```python
from build123d import *

# Parameters (mm, degrees)
BOSS_EXTRUDE1_DEPTH = 12.7
CUT_EXTRUDE1_DEPTH  = 25.4
CUT_EXTRUDE2_DEPTH  = 25.4
FILLET1_R           = 8.89
SKETCH4_R           = 2.54
CUT_EXTRUDE3_DEPTH  = 25.4


with BuildPart() as part:
    # Sketch1 → Boss-Extrude1 (new, symmetric)
    with BuildSketch(Plane.XY):
        Polygon((-19.05, 0), (19.05, 0), (19.05, -1.5875), (0, -3.175), (0, -1.5875), (-19.05, -1.5875), align=None)
    extrude(amount=BOSS_EXTRUDE1_DEPTH, both=True)

    # Sketch2 → Cut-Extrude1 (cut)
    with BuildSketch(Plane(origin=(0, 0, 0), x_dir=(1, 0, 0), z_dir=(0, 1, 0))):
        Polygon((0, 12.7), (19.05, 10.16), (19.05, 12.7), align=None)
    cut_extrude1 = extrude(amount=-CUT_EXTRUDE1_DEPTH, mode=Mode.SUBTRACT)

    # Mirror1: Cut-Extrude1 across plane
    add(cut_extrude1.mirror(Plane.XY), mode=Mode.SUBTRACT)

    # Sketch3 → Cut-Extrude2 (cut)
    with BuildSketch(Plane(origin=(0, 0, 0), x_dir=(1, 0, 0), z_dir=(0, 1, 0))):
        Polygon((0, 12.7), (-19.05, 7.62), (-19.05, 12.7), align=None)
    cut_extrude2 = extrude(amount=-CUT_EXTRUDE2_DEPTH, mode=Mode.SUBTRACT)

    # Mirror2: Cut-Extrude2 across plane
    add(cut_extrude2.mirror(Plane.XY), mode=Mode.SUBTRACT)

    # Fillet1
    fillet1_edges = [part.edges().sort_by_distance(p)[0] for p in [
        (-19.05, -0.79375, -7.62),
        (-19.05, -0.79375, 7.62),
    ]]
    fillet(fillet1_edges, radius=FILLET1_R)

    # Sketch4 → Cut-Extrude3 (cut)
    with BuildSketch(Plane(origin=(0, 0, 0), x_dir=(1, 0, 0), z_dir=(0, 1, 0))):
        with Locations(Location((-5.08, 5.543370255, 0), (0, 0, 270))):
            Circle(SKETCH4_R)
        with Locations(Location((-5.08, -5.837708499, 0), (0, 0, 270))):
            Circle(SKETCH4_R)
        with Locations(Location((-12.7, 0, 0), (0, 0, 270))):
            Circle(SKETCH4_R)
    extrude(amount=-CUT_EXTRUDE3_DEPTH, mode=Mode.SUBTRACT)


solid = part.part
```
Source: CAD feature listing. Evaluate the final solid. Frame: model axes, mm. A direction names the side the tool comes from. Round coordinates to 2 decimals unless told otherwise and drop trailing zeros. Order: outer loops, then holes, each group sorted by start corner. A loop starts at its lowest first (then second) coordinate and runs counter-clockwise, first axis right, second up. Notation, with made-up numbers: (-30.75, 6.5) -> (-6.75, 6.5) arc R13 ccw to (-6.75, 10.5) -> close; hole circle Ø2 at (-13.5, 5.25). An arc over 180 degrees is marked (long way). One line per item, written item: value. Start each with the question number.
Q1. Section query A-A (y = -0.7). Return the cut outline in (x, z), plus the area to 3 significant figures.
Q2. Pin query (flat end, axial travel): pin 1 (9.5 mm diameter, centred on x = -7.5, z = 6, fed in from -Y); pin 2 (1.5 mm diameter, centred on x = 10.5, z = 3, fed in from -Y); pin 3 (1.3 mm diameter, centred on y = -2.5, z = -4.5, fed in from -X). Return the tip coordinate at first contact, or that it passes through.
Q3. Material intervals for probe 1 along X at (y, z) = (-0.6, 0); probe 2 along X at (y, z) = (-0.2, -4.75); probe 3 along Y at (x, z) = (-1.5, -10.25), sorted ascending.
Q4. Access query for faces 5 (the flat face through (-7, -1.588, 0)), 6 (the flat face through (9.39, -1.21, -11.45)). Directions: +Z, -Z, +X, -X, +Y, -Y. A direction counts if a zero-diameter tool reaches every point of the face in a straight line with its end or side. Return the directions, or none.
Q5. Draft query along Z for faces 1 (the flat face through (-6.138, -0.783, 11.063)), 2 (the flat face through (-6.138, -0.783, -11.063)), 3 (the cylindrical face through (-4.32, -0.78, 8.26)), 4 (the cylindrical face through (-15.18, -0.78, -0.55)). Return one class per face: pulls with the +Z half, pulls with the -Z half, needs draft (parallel to the pull), parting line crosses it, or undercut.
Q6. Section query C-C (x = -5.08). Return the cut outline in (y, z), plus the area to 3 significant figures.
Findings below:
1. outline: (-19.05, -0.79) arc R8.89 ccw to (-12.45, -9.38) -> (0, -12.7) -> (19.05, -10.16) -> (19.05, 10.16) -> (0, 12.7) -> (-12.45, 9.38) arc R8.89 ccw to (-19.05, 0.79) -> close; hole circle Ø5.08 at (-12.7, 0); hole circle Ø5.08 at (-5.08, -5.54); hole circle Ø5.08 at (-5.08, 5.84)
1. area: 744 mm²
2. pin 1: y = -1.59
2. pin 2: y = -2.36
2. pin 3: x = 0
3. probe 1: -19.05 to -15.24, -10.16 to 19.05
3. probe 2: -18.12 to -7.49, -2.67 to 19.05
3. probe 3: -1.59 to 0
4. face 5: +Z, -Z, -X, -Y
4. face 6: -Z, +X, +Y, -Y
5. face 1: pulls with the +Z half
5. face 2: pulls with the -Z half
5. face 3: undercut
5. face 4: undercut
6. outline: (-1.59, -11.35) -> (0, -11.35) -> (0, -8.08) -> (-1.59, -8.08) -> close; (-1.59, -3) -> (0, -3) -> (0, 3.3) -> (-1.59, 3.3) -> close; (-1.59, 8.38) -> (0, 8.38) -> (0, 11.35) -> (-1.59, 11.35) -> close
6. area: 19.9 mm²
